Here's how the part is built. I have some questions about the finished solid (model axes, mm). Face numbers are marked on the shaded views. A direction names the side the tool comes from. Coordinates: 2 decimals unless noted, no trailing zeros. Write each loop counter-clockwise with the first axis right and the second up, starting at its lowest first coordinate (ties: lowest second). Pieces come first, ordered by that corner, then holes.
(1) For pin 1 Ø1.5 at (x, z) = (7.5, 3.5) entering from +Y; pin 2 Ø6 at (x, z) = (6.5, 5.5) entering from +Y; pin 3 Ø1.5 at (y, z) = (8.5, 2.5) entering from +X, each with a flat end and sliding along its axis, tell me the tip position at first contact or that it passes through.
(2) Imagine slicing it at A-A, the plane z = 0. List the corners of the cut face in (x, y) for me, plus the area to 4 significant figures.
(3) Please list where these lines run through material, in increasing order: probe 1 along Y at (x, z) = (1.05, 0); probe 2 along Z at (x, y) = (1.25, 1.25); probe 3 along X at (y, z) = (4.75, -3).
(4) Imagine slicing it at C-C, the plane z = 9. List the corners of the cut face in (x, y) for me, plus the area to 3 significant figures.
(5) Imagine slicing it at D-D, the plane y = 6.75. List the corners of the cut face in (x, z) for me.
(6) Which directions (+Z, -Z, +X, -X, +Y, -Y) give clear straight access to the entire face, cutting with the end or side of a thin tool? Please do the marked faces 1, 2 and 3.
(7) Thinking about a two-plate mould opening in Z: for the marked faces 4, 5 and 6, which applies, released by +Z, released by -Z, zero draft, split by the parting line, or undercut?
```python
from build123d import *

# Parameters (mm, degrees)
CROQUIS1_R              = 11
CROQUIS1_R_2            = 1.75
SALIENTE_EXTRUIR1_DEPTH = 3
CROQUIS2_R              = 5.1
SALIENTE_EXTRUIR2_DEPTH = 10
CHAFL_N1_SIZE           = 0.5
SALIENTE_EXTRUIR3_START = 1.5
CROQUIS3_R              = 5.1
SALIENTE_EXTRUIR3_DEPTH = 1.5
CROQUIS4_R              = 4
CORTAR_EXTRUIR1_DEPTH   = 22.266170318


with BuildPart() as part:
    # Croquis1 → Saliente-Extruir1 (new body)
    with BuildSketch(Plane(origin=(0, 0, 0), x_dir=(0, 0, -1), z_dir=(1, 0, 0))):
        Circle(CROQUIS1_R)
        with Locations((0, 8)):
            Circle(CROQUIS1_R_2, mode=Mode.SUBTRACT)
        with Locations((8, 0)):
            Circle(CROQUIS1_R_2, mode=Mode.SUBTRACT)
        with Locations((0, -8)):
            Circle(CROQUIS1_R_2, mode=Mode.SUBTRACT)
        with Locations((-8, 0)):
            Circle(CROQUIS1_R_2, mode=Mode.SUBTRACT)
    extrude(amount=SALIENTE_EXTRUIR1_DEPTH)

    # Croquis2 → Saliente-Extruir2 (add)
    with BuildSketch(Plane(origin=(3, 0, 0), x_dir=(0, 0, -1), z_dir=(1, 0, 0))):
        Circle(CROQUIS2_R)
    extrude(amount=SALIENTE_EXTRUIR2_DEPTH)

    # Chaflán1
    chafl_n1_edges = [part.edges().sort_by_distance(p)[0] for p in [
        (13, 0, 5.1),
    ]]
    chamfer(chafl_n1_edges, length=CHAFL_N1_SIZE)

    # Croquis3 → Saliente-Extruir3 (add)
    with BuildSketch(Plane.ZY.offset(SALIENTE_EXTRUIR3_START)):
        with Locations(Location((0, 0, 0), (0, 0, 180))):
            Circle(CROQUIS3_R)
    extrude(amount=-SALIENTE_EXTRUIR3_DEPTH)

    # Croquis4 → Cortar-Extruir1 (cut, through all)
    with BuildSketch(Plane(origin=(13, 0, 0), x_dir=(0, 0, -1), z_dir=(1, 0, 0))):
        Circle(CROQUIS4_R)
    extrude(amount=-CORTAR_EXTRUIR1_DEPTH, mode=Mode.SUBTRACT)


solid = part.part
```
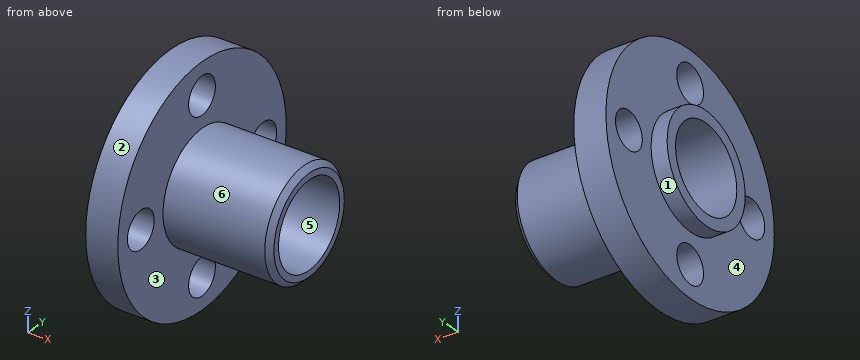
Recorded:
1. pin 1: stops at y = 4.3
1. pin 2: stops at y = 4.45
1. pin 3: stops at x = 3
2. outline: (-1.5, -5.1) - (0, -5.1) - (0, -6.25) - (3, -6.25) - (3, -5.1) - (12.5, -5.1) - (13, -4.6) - (13, -4) - (-1.5, -4) - close; (-1.5, 4) - (13, 4) - (13, 4.6) - (12.5, 5.1) - (3, 5.1) - (3, 6.25) - (0, 6.25) - (0, 5.1) - (-1.5, 5.1) - close; (0, -11) - (3, -11) - (3, -9.75) - (0, -9.75) - close; (0, 9.75) - (3, 9.75) - (3, 11) - (0, 11) - close
2. area: 46.05 mm2
3. probe 1: y = -11 to -9.75, -6.25 to -4, 4 to 6.25, 9.75 to 11
3. probe 2: z = -10.93 to -9.22, -6.78 to -3.8, 3.8 to 6.78, 9.22 to 10.93
3. probe 3: x = 0 to 3
4. outline: (0, -6.32) - (3, -6.32) - (3, -1.44) - (0, -1.44) - close; (0, 1.44) - (3, 1.44) - (3, 6.32) - (0, 6.32) - close
4. area: 29.3 mm2
5. outline: (0, -8.69) - (3, -8.69) - (3, -1.22) - (0, -1.22) - close; (0, 1.22) - (3, 1.22) - (3, 8.69) - (0, 8.69) - close
6. face 1: -X
6. face 2: +X, -X
6. face 3: +X
7. face 4: zero draft
7. face 5: undercut
7. face 6: split by the parting line
